Autodesk Inventor part; units mm, degrees
ref_plane "YZ Plane" through (0, 0, 0) normal (1, 0, 0) x (0, 1, 0)
ref_plane "XZ Plane" through (0, 0, 0) normal (0, 1, 0) x (-1, 0, 0)
ref_plane "XY Plane" through (0, 0, 0) normal (0, 0, 1) x (1, 0, 0)
sketch "Sketch1" plane through (0, 0, 0) normal (0, 0, 1) x (1, 0, 0)
  line L0 (-45, 35) -> (50, 35)
  line L1 (50, 35) -> (50, -35)
  line L2 (50, -35) -> (-45, -35)
  line L3 (-45, -35) -> (-45, 35)
  line L4 (-38.5, 26.5) -> (38.5, 26.5) construction
  line L5 (38.5, 26.5) -> (38.5, -26.5) construction
  line L6 (38.5, -26.5) -> (-38.5, -26.5) construction
  line L7 (-38.5, -26.5) -> (-38.5, 26.5) construction
  circle A0 centre (-38.5, 26.5) radius 2.5
  circle A1 centre (38.5, 26.5) radius 2.5
  circle A2 centre (38.5, -26.5) radius 2.5
  circle A3 centre (-38.5, -26.5) radius 2.5
  line L8 (-30, 27.5) -> (30, 27.5)
  line L9 (30, 27.5) -> (30, -27.5)
  line L10 (30, -27.5) -> (-30, -27.5)
  line L11 (-30, -27.5) -> (-30, 27.5)
  line L12 (30, 15) -> (40, 15)
  line L13 (40, 15) -> (40, -15)
  line L14 (40, -15) -> (30, -15)
  line L15 (30, -15) -> (30, 15)
  line L16 (-30, 15) -> (-40, 15)
  line L17 (-40, 15) -> (-40, -15)
  line L18 (-40, -15) -> (-30, -15)
  line L19 (-30, -15) -> (-30, 15)
  point P0 (0, 0)
  point P1 (50, 0)
  point P2 (2.5, 35)
  point P3 (38.5, 0)
  point P4 (0, 26.5)
  point P5 (30, 0)
  point P6 (0, 27.5)
  point P7 (-40, 0)
  point P8 (40, 0)
  dimension "d1" = 70
  dimension "d2" = 77
  dimension "d3" = 53
  dimension "d14" = 5
  dimension "d23" = 45
  dimension "d24" = 50
  dimension "d25" = 55
  dimension "d26" = 60
  dimension "d27" = 30
  dimension "d28" = 10
  dimension "d29" = 10
extrude "Extrusion1" add sketch "Sketch1" along normal blind 3 contours L0 L1 L2 L3 | A0 | A1 | A2 | A3
hole "Hole1" at (38.5, 26.5, 0) at (38.5, -26.5, 0) at (-38.5, -26.5, 0) at (-38.5, 26.5, 0) direction (0, 0, 1) diameter 4 end through all
fillet "Fillet1" radius 5 16 edges at (50, 35, 1.5) (50, -35, 1.5) (-45, -35, 1.5) (-45, 35, 1.5) (-30, 27.5, 1.5) (30, 27.5, 1.5) (30, -27.5, 1.5) (-30, -27.5, 1.5) (-30, 15, 1.5) (-40, 15, 1.5) (-40, -15, 1.5) (-30, -15, 1.5) (30, 15, 1.5) (40, 15, 1.5) (40, -15, 1.5) (30, -15, 1.5)
chamfer "Chamfer2" distance 0.5 angle 45 44 edges at (2.5, 35, 0) (-43.5357, 33.5357, 0) (-45, 0, 0) (-43.5357, -33.5357, 0) (2.5, -35, 0) (48.5357, -33.5357, 0) (50, 0, 0) (48.5357, 33.5357, 0) (2.5, 35, 3) (-43.5357, 33.5357, 3) (-45, 0, 3) (-43.5357, -33.5357, 3) (2.5, -35, 3) (48.5357, -33.5357, 3) (50, 0, 3) (48.5357, 33.5357, 3) (0, 27.5, 3) (31.4643, 16.4643, 3) (35, 15, 3) (40, 0, 3) (35, -15, 3) (31.4643, -16.4643, 3) (0, -27.5, 3) (-30, -21.25, 3) (-31.4643, -16.4643, 3) (-35, -15, 3) (-40, 0, 3) (-35, 15, 3) (-31.4643, 16.4643, 3) (-30, 21.25, 3) (0, 27.5, 0) (31.4643, 16.4643, 0) (35, 15, 0) (40, 0, 0) (35, -15, 0) (31.4643, -16.4643, 0) (0, -27.5, 0) (-30, -21.25, 0) (-31.4643, -16.4643, 0) (-35, -15, 0) (-40, 0, 0) (-35, 15, 0) (-31.4643, 16.4643, 0) (-30, 21.25, 0)
chamfer "Chamfer3" distance 0.4 angle 45 8 edges at (-38.5, -28.5, 3) (38.5, -28.5, 3) (-38.5, 24.5, 3) (38.5, 24.5, 3) (-38.5, -28.5, 0) (38.5, -28.5, 0) (-38.5, 24.5, 0) (38.5, 24.5, 0)
equation "\"d1\" = width"
equation "\"d4\" = thickness"
equation "\"width\" = 70"
equation "\"thickness\" = 3"
equation "\"bump\" = 3"
properties part number "temp-logger-base-plate-v2" material "ABS Plastic"
For this review, take the finished solid that the model builds, in its own axes (mm). A direction names the side the tool comes from. Coordinates: 2 decimals unless noted, no trailing zeros. Loops run counter-clockwise (first coordinate to the right, second up) from the corner with the lowest first, then second, coordinate; pieces in that order, holes last.
1. For line 1 (X direction, y = 26.5, z = 1.05); line 2 (Y direction, x = 4, z = 0.85); line 3 (Y direction, x = 39.5, z = 0.7), list the stretches that pass through material, from the lowest coordinate up.
2. Add section A-A, the plane y = -9. Give the boundary of the cut face in (x, z).
3. Add section B-B, the plane x = 15. Give the boundary of the cut face in (y, z), then the cut area to 3 significant figures.
4. Mouldability with a two-part tool opening along Y and no side actions: class faces 1 (the cylindrical face through (-31, -17, 2)), 2 (the conical face through (-43.319, -33.247, 0.142)), 3 (the flat face through (50, 0, 1)), 4 (the flat face through (-40, 0, 1)) as +Y half, -Y half, draft (parallel to the pull), parting line (faces both ways), or undercut.
5. Add section C-C, the plane z = 1.7. Count the separate pieces of the cut face and the enclosed holes in it, then the cut area to 3 significant figures.
6. Insertion check: P1, Ø2.5, axis at x = 38.5, y = 26.5, coming from the -Z side; P2, Ø4.5, axis at x = 38.5, y = -26.5, coming from the +Z side; P3, Ø5, axis at x = -38.5, y = 26.5, coming from the +Z side. Each pin has a flat end and moves straight along its axis. Give the tip position at first contact, or say it passes through.
7. For faces 5 (the conical face through (-31.753, 16.681, 0.142)), 6 (the conical face through (-43.247, 33.319, 0.142)), 7 (the cylindrical face through (39, 13, 2)), 8 (the conical face through (28.676, 26.096, 2.642)), list the 3-axis set-ups (+Z, -Z, +X, -X, +Y, -Y) from which the entire face can be reached by the end or side of a thin tool; tool diameter is ignored.
Result:
1. line 1: x = -45 to -40.5, -36.5 to -28, 28 to 36.5, 40.5 to 50
1. line 2: y = -35 to -27.5, 27.5 to 35
1. line 3: y = -35 to -28.23, -24.77 to -12.18, 12.18 to 24.77, 28.23 to 35
2. outline: (-45, 0.5) - (-44.5, 0) - (-40.5, 0) - (-40, 0.5) - (-40, 2.5) - (-40.5, 3) - (-44.5, 3) - (-45, 2.5) - close; (40, 0.5) - (40.5, 0) - (49.5, 0) - (50, 0.5) - (50, 2.5) - (49.5, 3) - (40.5, 3) - (40, 2.5) - close
3. outline: (-35, 0.5) - (-34.5, 0) - (-28, 0) - (-27.5, 0.5) - (-27.5, 2.5) - (-28, 3) - (-34.5, 3) - (-35, 2.5) - close; (27.5, 0.5) - (28, 0) - (34.5, 0) - (35, 0.5) - (35, 2.5) - (34.5, 3) - (28, 3) - (27.5, 2.5) - close
3. area: 44.0 mm2
4. face 1: undercut
4. face 2: -Y half
4. face 3: draft
4. face 4: undercut
5. separate pieces: 1
5. enclosed holes: 5
5. area: 2,700 mm2
6. P1: passes through
6. P2: stops at z = 2.85
6. P3: stops at z = 3
7. face 5: -Z
7. face 6: -Z, -X, +Y
7. face 7: +Z, -Z
7. face 8: +Z
